Autodesk Inventor part; units mm, degrees
ref_plane "YZ Plane" through (0, 0, 0) normal (1, 0, 0) x (0, 1, 0)
ref_plane "XZ Plane" through (0, 0, 0) normal (0, 1, 0) x (-1, 0, 0)
ref_plane "XY Plane" through (0, 0, 0) normal (0, 0, 1) x (1, 0, 0)
ref_plane "Work Plane1" through (0, 0, 0) normal (0, 0, 1) x (1, 0, 0)
sketch "Sketch1" plane through (0, 0, 0) normal (0, 0, 1) x (1, 0, 0)
  line L0 (-17.825, 16.8) -> (-17.825, -16.8) construction
  line L1 (-17.825, -16.8) -> (-7, -16.8) construction
  line L2 (-7, -16.8) -> (-7, -13.05) construction
  line L3 (-7, -13.05) -> (7, -13.05) construction
  line L4 (7, -13.05) -> (7, -16.8) construction
  line L5 (7, -16.8) -> (17.825, -16.8) construction
  line L6 (17.825, -16.8) -> (17.825, 16.8) construction
  line L7 (17.825, 16.8) -> (-17.825, 16.8) construction
  circle A0 centre (15.24, 13.97) radius 2.5 construction
  circle A1 centre (-15.24, 13.97) radius 2.5 construction
  circle A2 centre (-15.24, -13.97) radius 2.5 construction
  circle A3 centre (15.24, -13.97) radius 2.5 construction
  line L8 (-18.825, 17.8) -> (-7.08, 17.8)
  line L9 (-7.08, 17.8) -> (-7.08, 11.8)
  line L10 (-7.08, 11.8) -> (7.08, 11.8)
  line L11 (7.08, 11.8) -> (7.08, 17.8)
  line L12 (7.08, 17.8) -> (18.825, 17.8)
  line L13 (18.825, 17.8) -> (18.825, -17.8)
  line L14 (18.825, -17.8) -> (-18.825, -17.8)
  line L15 (-18.825, -17.8) -> (-18.825, 17.8)
  line L16 (-5.08, 14.5) -> (-5.08, 16.3)
  line L17 (5.08, 14.5) -> (5.08, 16.3)
  point P0 (0, 0)
  dimension "d0" = 1
  dimension "d1" = 1
  dimension "d2" = 1
  dimension "d3" = 1
  dimension "d4" = 2
  dimension "d5" = 5
extrude "Extrusion1" add sketch "Sketch1" along normal blind 5
sketch "Sketch2" plane through (0, 0, 5) normal (0, 0, 1) x (1, 0, 0)
  circle A0 centre (-15.24, 13.97) radius 1.5
  circle A1 centre (-15.24, -13.97) radius 1.5
  circle A2 centre (15.24, -13.97) radius 1.5
  circle A3 centre (15.24, 13.97) radius 1.5
  point P0 (0, 0)
extrude "Extrusion2" cut sketch "Sketch2" against normal blind 3
sketch "Sketch3" plane through (0, 0, 0) normal (0, 0, -1) x (-1, 0, 0)
  circle A0 centre (-15.24, 13.97) radius 1.5 construction
  circle A1 centre (15.24, 13.97) radius 1.5 construction
  circle A2 centre (15.24, -13.97) radius 1.5 construction
  circle A3 centre (-15.24, -13.97) radius 1.5 construction
  circle A4 centre (-15.24, 13.97) radius 1.45
  circle A5 centre (15.24, 13.97) radius 1.45
  circle A6 centre (15.24, -13.97) radius 1.45
  circle A7 centre (-15.24, -13.97) radius 1.45
  point P0 (0, 0)
  dimension "d10" = 2.9
extrude "Extrusion3" add sketch "Sketch3" along normal blind 2 contours A4 | A5
sketch "Sketch4" plane through (0, 0, 0) normal (0, 0, -1) x (-1, 0, 0)
  line L0 (18.825, 17.8) -> (18.825, -17.8)
  line L1 (7.08, 17.8) -> (18.825, 17.8)
  line L2 (-18.825, 17.8) -> (-7.08, 17.8)
  line L3 (-18.825, -17.8) -> (-18.825, 17.8)
  line L4 (18.825, -17.8) -> (-18.825, -17.8)
  line L5 (7.08, 11.8) -> (7.08, 17.8)
  line L6 (7.08, 17.8) -> (7.08, 17.3)
  line L7 (7.08, 17.3) -> (18.325, 17.3)
  line L8 (18.325, 17.3) -> (18.325, -17.3)
  line L9 (18.325, -17.3) -> (-18.325, -17.3)
  line L10 (-18.325, -17.3) -> (-18.325, 17.3)
  line L11 (-18.325, 17.3) -> (-7.08, 17.3)
  line L12 (-7.08, 17.3) -> (-7.08, 17.8)
  line L13 (-18.325, -17.3) -> (-18.325, -17.8)
  line L14 (18.325, -17.3) -> (18.325, -17.8)
  line L15 (18.825, -17.8) -> (-18.825, -17.8)
  point P0 (0, 0)
  dimension "d13" = 0.5
  dimension "d14" = 0.5
  dimension "d15" = 0.5
  dimension "d16" = 0.5
extrude "Extrusion4" add sketch "Sketch4" along normal blind 2 contours L0 L4 L14 L8 L7 L5 L1 | L4 L3 L2 L12 L11 L10 L13
sketch "Sketch5" plane through (7.08, 17.8, 5) normal (0, 1, 0) x (1, 0, 0)
  line L0 (23.7251, 17.6627) -> (-33.6889, 17.6627)
  line L1 (-33.6889, 17.6627) -> (-33.6889, -9.8348)
  line L2 (-33.6889, -9.8348) -> (23.7251, -9.8348)
  line L3 (23.7251, -9.8348) -> (23.7251, 17.6627)
  point P0 (-7.08, 5)
extrude "Extrusion5" cut sketch "Sketch5" against normal blind 2
sketch "Sketch6" plane through (0, 0, 0) normal (0, 0, -1) x (-1, 0, 0)
  line L0 (-17.325, 11.8) -> (17.325, 11.8)
  line L1 (17.325, 11.8) -> (17.325, -14.8)
  line L2 (17.325, -14.8) -> (-17.325, -14.8)
  line L3 (-17.325, -14.8) -> (-17.325, 11.8)
  line L4 (-7.08, 11.8) -> (7.08, 11.8)
  line L5 (-18.325, -17.8) -> (-18.325, 15.8)
  line L6 (18.325, 15.8) -> (18.325, -17.8)
  line L7 (18.325, -17.8) -> (-18.325, -17.8)
  point P0 (0, 0)
  point P1 (0, 11.8)
  dimension "d21" = 1
  dimension "d22" = 1
  dimension "d23" = 3
extrude "Extrusion6" cut sketch "Sketch6" against normal blind 1.5
properties part number "OledCarrier"
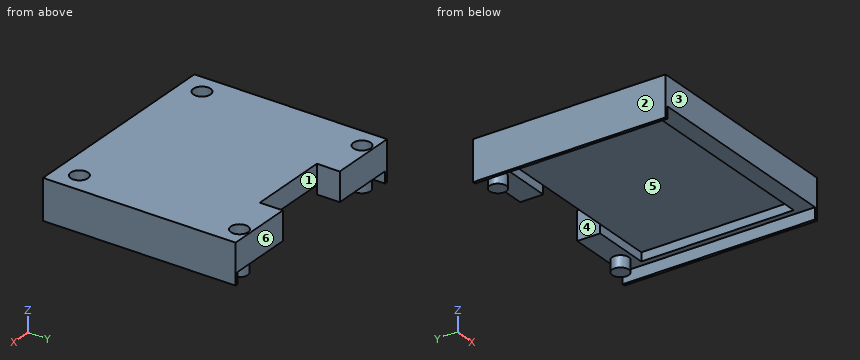
Source: CAD feature listing. Evaluate the final solid. Frame: model axes, mm. Face numbers are marked on the shaded views. A direction names the side the tool comes from. Coordinates: 2 decimals unless noted, no trailing zeros. Order: outer loops, then holes, each group sorted by start corner. A loop starts at its lowest first (then second) coordinate and runs counter-clockwise, first axis right, second up. Notation, with made-up numbers: M 46,-3 L 57,-3 A18 cw 57,2 Z; hole C -13,25 d8. An arc over 180 degrees is marked long. Write each question's results on one line, items separated by ' | '. Start each with the question number.
1) Access query for the marked faces 1 and 2. Directions: +Z, -Z, +X, -X, +Y, -Y. A direction counts if a zero-diameter tool reaches every point of the face in a straight line with its end or side. Return the directions, or none.
2) Section query A-A (z = -1). Return the cut outline in (x, y) (3 decimals), plus the area to 3 significant figures.
3) Section query B-B (y = 13.97). Return the cut outline in (x, z) (3 decimals), plus the area to 3 significant figures.
4) Section query C-C (z = 3.75). Return the cut outline in (x, y) (3 decimals), plus the area to 3 significant figures.
5) Contact query for flat-ended pins moving along their axis: pin 1 Ø1.5 at (x, y) = (15.5, -14) entering from +Z; pin 2 Ø0.8 at (x, z) = (-2, 0.5) entering from +Y; pin 3 Ø2 at (x, y) = (1, 12.5) entering from -Z. Output: stop coordinate, or through.
6) Draft query along Y for the marked faces 3, 4, 5 and 6. Return one class per face: released by +Y, released by -Y, zero draft, split by the parting line, or undercut.
7) Section query D-D (y = -10.5). Return the cut outline in (x, z) (3 decimals).
8) Line query: line 1 (Y direction, x = -15.24, z = 3.85); line 2 (X direction, y = 11, z = -1) (3 decimals); line 3 (Z direction, x = 7.5, y = -15). Output: solid intervals per line, ascending. Write a range as from..to.
Answers:
1) face 1: +Z, -Z, +Y | face 2: +Z, -Z, -X, +Y, -Y
2) outline: M -18.825,-17.8 L -18.325,-17.8 L -18.325,15.8 L -18.825,15.8 Z; C -15.24,13.97 d2.9; C 15.24,13.97 d2.9; M 18.325,-17.8 L 18.825,-17.8 L 18.825,15.8 L 18.325,15.8 Z | area: 46.8 mm^2
3) outline: M -18.825,-2 L -18.325,-2 L -18.325,0 L -16.69,0 L -16.69,-2 L -13.79,-2 L -13.79,0 L -7.08,0 L -7.08,5 L -13.74,5 L -13.74,2 L -16.74,2 L -16.74,5 L -18.825,5 Z; M 7.08,0 L 13.79,0 L 13.79,-2 L 16.69,-2 L 16.69,0 L 18.325,0 L 18.325,-2 L 18.825,-2 L 18.825,5 L 16.74,5 L 16.74,2 L 13.74,2 L 13.74,5 L 7.08,5 Z | area: 113 mm^2
4) outline: M -18.825,-17.8 L 18.825,-17.8 L 18.825,15.8 L 7.08,15.8 L 7.08,11.8 L -7.08,11.8 L -7.08,15.8 L -18.825,15.8 Z; hole C -15.24,-13.97 d3; hole C -15.24,13.97 d3; hole C 15.24,-13.97 d3; hole C 15.24,13.97 d3 | area: 1,180 mm^2
5) pin 1: stops at z = 2 | pin 2: stops at y = -14.8 | pin 3: stops at z = 1.5
6) face 3: released by -Y | face 4: zero draft | face 5: undercut | face 6: released by +Y
7) outline: M -18.825,-2 L -18.325,-2 L -18.325,0 L -17.325,0 L -17.325,1.5 L 17.325,1.5 L 17.325,0 L 18.325,0 L 18.325,-2 L 18.825,-2 L 18.825,5 L -18.825,5 Z
8) line 1: y = -17.8..-15.47, -12.47..12.47, 15.47..15.8 | line 2: x = -18.825..-18.325, 18.325..18.825 | line 3: z = 0..5
